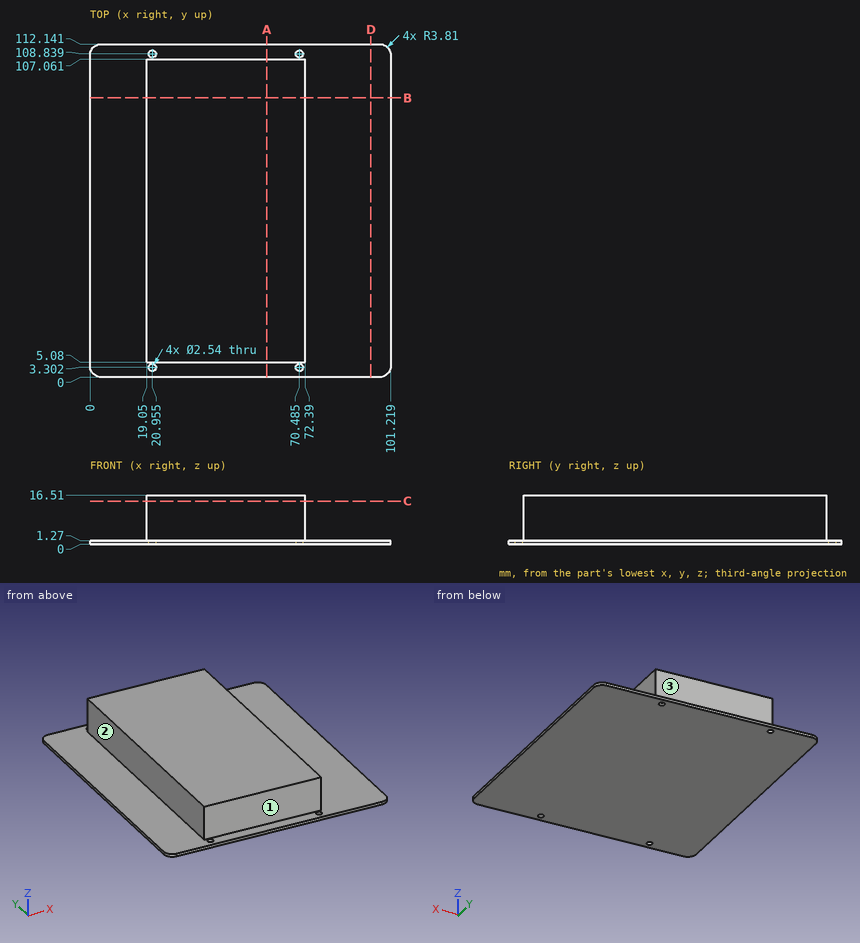
The drawing under review shows one solid part. Ordinate dimensions are in mm from its lowest x, y, z. A direction names the side the tool comes from. Give positions to 0.01 mm unless a question says otherwise; leave off trailing zeros. Write each loop counter-clockwise with the first axis right and the second up, starting at its lowest first coordinate (ties: lowest second). Pieces come first, ordered by that corner, then holes. Notation, with made-up numbers: (20, 88) - (69, 88) arc R6 cw to (69, 95) - close; hole circle Ø11 at (40, 6.5). An arc over 180 degrees is marked (long way). Answer in a Markdown table with one row per item. Add a question column.
1. We need section C-C on z = 14.5. Write out the cut boundary in (x, y).
2. Tool access review of the marked faces 1, 2 and 3: name each direction out of +Z, -Z, +X, -X, +Y, -Y from which nothing blocks a thin tool from reaching the whole face with its end or side.
3. We need section A-A on x = 59.5. Write out the cut boundary in (y, z).
4. Wall thickness on line 1 along Z through (x, y) = (94.5, 85); line 2 along X through (y, z) = (82, 6.75); line 3 along Y through (x, z) = (29.5, 6.75): over which ranges is each line inside the solid? List them lowest first. Write a range as [from, to].
5. Insertion check: P1, Ø8, axis at y = 34, z = 10, coming from the -X side; P2, Ø3, axis at x = 70.485, y = 3.302, coming from the -Z side; P3, Ø7.5, axis at x = 32.5, z = 10.5, coming from the +Y side; P4, Ø1, axis at x = 16.5, z = 3.5, coming from the +Y side (3 decimals). Each pin has a flat end and moves straight along its axis. Give the tip position at first contact, or say it passes through.
6. We need section D-D on x = 94.5. Write out the cut boundary in (y, z).
7. We need section B-B on y = 94. Write out the cut boundary in (x, z), then the cut area to 3 significant figures.
Ans:
| question | item | result |
|---|---|---|
| 1 | outline | (19.05, 5.08) - (72.39, 5.08) - (72.39, 107.06) - (19.05, 107.06) - close |
| 2 | face 1 | +Z, +X, -X, -Y |
| 2 | face 2 | +Z, -X, +Y, -Y |
| 2 | face 3 | +Z, +X, -X, +Y |
| 3 | outline | (0, 0) - (112.14, 0) - (112.14, 1.27) - (107.06, 1.27) - (107.06, 16.51) - (5.08, 16.51) - (5.08, 1.27) - (0, 1.27) - close |
| 4 | line 1 | z = [0, 1.27] |
| 4 | line 2 | x = [19.05, 72.39] |
| 4 | line 3 | y = [5.08, 107.06] |
| 5 | P1 | stops at x = 19.05 |
| 5 | P2 | stops at z = 0 |
| 5 | P3 | stops at y = 107.06 |
| 5 | P4 | passes through |
| 6 | outline | (0, 0) - (112.14, 0) - (112.14, 1.27) - (0, 1.27) - close |
| 7 | outline | (0, 0) - (101.22, 0) - (101.22, 1.27) - (72.39, 1.27) - (72.39, 16.51) - (19.05, 16.51) - (19.05, 1.27) - (0, 1.27) - close |
| 7 | area | 941 mm^2 |
